Geometry: final body of the model. Coordinates: model frame, mm. Face numbers are marked on the shaded views. A direction names the side the tool comes from. Round coordinates to 2 decimals unless told otherwise and drop trailing zeros. Loops run counter-clockwise (first coordinate to the right, second up) from the corner with the lowest first, then second, coordinate; pieces in that order, holes last. Notation, with made-up numbers: (-13, 79) - (-3, 79) arc R23 cw to (-3, 92) - close; hole circle Ø2 at (48, -36.75). An arc over 180 degrees is marked (long way). Answer as a JSON object with one key per item and string values. Group by question number.
Item 1: Draft query along Z for the marked faces 1, 2 and 3. Return one class per face: released by +Z, released by -Z, zero draft, split by the parting line, or undercut.
Item 2: First-contact query: pin 1 (10 mm diameter, centred on x = -59, y = 3, fed in from -Z); pin 2 (3.5 mm diameter, centred on x = -7.36, z = 4.25, fed in from +Y); pin 3 (8 mm diameter, centred on y = 3.5, z = -39.5, fed in from +X); pin 4 (1.8 mm diameter, centred on x = 0, z = -8.5, fed in from +Y). Flat tips, straight axial feed; report the tip coordinate or a pass-through.
Item 3: Section C-C (y = 6). Return the cut outline in (x, z), plus the area to 3 significant figures.
Item 4: Section D-D (z = -62). Return the cut outline in (x, y).
Item 5: Section A-A (x = 33). Return the cut outline in (y, z), plus the area to 3 significant figures.
Item 6: Section B-B (z = -34). Return the cut outline in (x, y), plus the area to 3 significant figures.
Item 7: Line query: line 1 (Z direction, x = 0, y = 17.05); line 2 (Z direction, x = 0, y = 23.75); line 3 (Z direction, x = 0, y = 15.95). Output: solid intervals per line, ascending.
Item 8: Reachability of the marked faces 4 and 5 from +Z, -Z, +X, -X, +Y, -Y: full face, straight path, thin tool, end or side. Return the list, or none.
Autodesk Inventor part; units mm, degrees
ref_plane "YZ Plane" through (0, 0, 0) normal (1, 0, 0) x (0, 1, 0)
ref_plane "XZ Plane" through (0, 0, 0) normal (0, 1, 0) x (-1, 0, 0)
ref_plane "XY Plane" through (0, 0, 0) normal (0, 0, 1) x (1, 0, 0)
sketch "Sketch1" plane through (0, 0, 0) normal (0, 0, 1) x (1, 0, 0)
  line L0 (0, 20) -> (75, 20)
  line L1 (75, 20) -> (75, 0)
  line L2 (75, 0) -> (60, 0)
  line L3 (60, 0) -> (60, 14)
  line L4 (60, 14) -> (0, 14)
  line L5 (0, 14) -> (0, 20)
  line L6 (-15, 0) -> (90, 0)
  line L7 (0, -4) -> (0, 24)
  point P0 (0, 0)
  dimension "d2" = 14
  dimension "d3" = 20
  dimension "d5" = 150
  dimension "d6" = 120
revolve "Revolution1" add sketch "Sketch1" angle 360 about axis through (0, 14, 0) along (0, 1, 0) contours L0 L1 L2 L3 L4 L5
sketch "Sketch2" plane through (0, 20, 0) normal (0, 1, 0) x (1, 0, 0)
  circle A0 centre (0, 0) radius 75
  circle A1 centre (0, 0) radius 2
  dimension "d7" = 4
extrude "Extrusion1" cut sketch "Sketch2" against normal through all contours A1
sketch "Sketch3" plane through (0, 20, 0) normal (0, 1, 0) x (1, 0, 0)
  circle A0 centre (0, 0) radius 2
  line L0 (0, 105) -> (0, -105)
  line L1 (-105, 0) -> (105, 0)
  point P0 (0, 8.5)
  point P1 (-7.3612, -4.25)
  point P2 (7.3612, -4.25)
  dimension "d10" = 8.5
  dimension "d13" = 360
hole "Hole1" at (0, 20, -8.5) at (-7.3612, 20, 4.25) at (7.3612, 20, 4.25) direction (0, -1, 0) diameter 3 end through all
sketch "Sketch4" plane through (0, 20, 0) normal (0, 1, 0) x (1, 0, 0)
  circle A0 centre (0, 0) radius 22.5
  circle A1 centre (0, 0) radius 25.5
  circle A2 centre (0, 0) radius 19.5
  dimension "d23" = 45
  dimension "d24" = 3
  dimension "d25" = 3
extrude "Extrusion2" add sketch "Sketch4" along normal blind 7 contours A0 | A1
sketch "Sketch5" plane through (0, 27, 0) normal (0, 1, 0) x (1, 0, 0)
  circle A0 centre (0, 0) radius 22.5
  point P0 (-22.5, 0)
  point P1 (0, -22.5)
  point P2 (22.5, 0)
  point P3 (0, 22.5)
  dimension "d28" = 45
hole "Hole2" at (-22.5, 27, 0) at (0, 27, 22.5) at (22.5, 27, 0) at (0, 27, -22.5) direction (0, -1, 0) diameter 2.459 depth 10 tip angle 118
properties part number "Wheel 2" material "Brass, Soft Yellow, Welded"
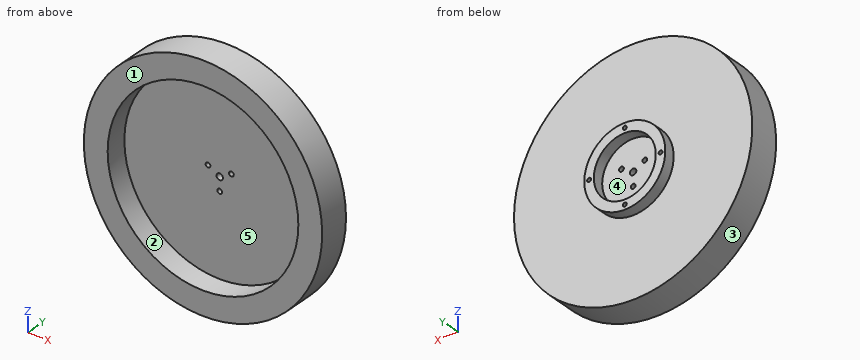
Values:
{
 "1": {"face 1": "zero draft", "face 2": "undercut", "face 3": "split by the parting line"},
 "2": {"pin 1": "stops at z = -52.05", "pin 2": "stops at y = 20", "pin 3": "stops at x = 66.07", "pin 4": "passes through"},
 "3": {"outline": "circle Ø150 at (0, 0); hole circle Ø120 at (0, 0)", "area": "6,360 mm^2"},
 "4": {"outline": "(-42.2, 0) - (42.2, 0) - (42.2, 20) - (-42.2, 20) - close"},
 "5": {"outline": "(0, -67.35) - (20, -67.35) - (20, 67.35) - (0, 67.35) - (0, 50.11) - (14, 50.11) - (14, -50.11) - (0, -50.11) - close", "area": "1,290 mm^2"},
 "6": {"outline": "(-66.85, 0) - (-49.44, 0) - (-49.44, 14) - (49.44, 14) - (49.44, 0) - (66.85, 0) - (66.85, 20) - (-66.85, 20) - close", "area": "1,290 mm^2"},
 "7": {"line 1": "z = -75 to -23.73, -21.27 to -10, -7 to -2, 2 to 21.27, 23.73 to 75", "line 2": "z = -25.5 to -23.73, -21.27 to -19.5, 19.5 to 21.27, 23.73 to 25.5", "line 3": "z = -75 to -10, -7 to -2, 2 to 75"},
 "8": {"face 4": "+Y", "face 5": "-Y"}
}
